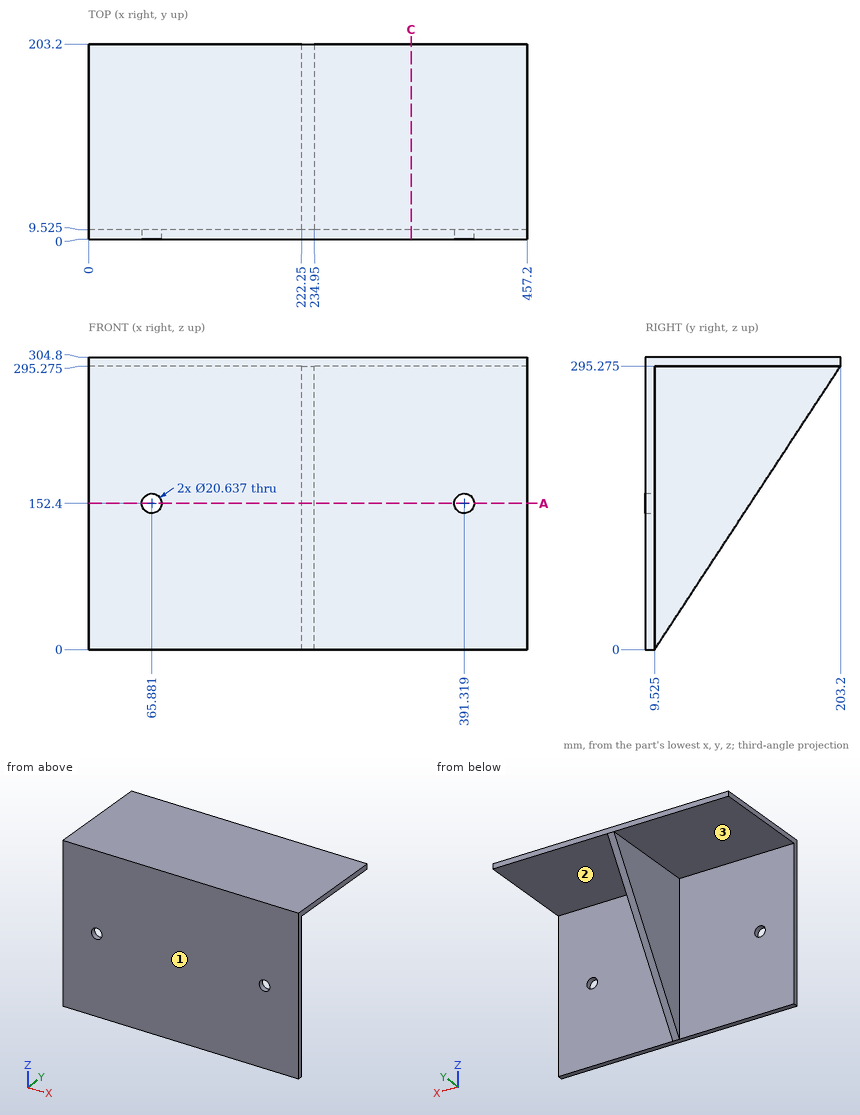
Verification items for this drawing (mm, ordinates from the low corner). A direction names the side the tool comes from. Give positions to 0.01 mm unless a question says otherwise; leave off trailing zeros. Order: outer loops, then holes, each group sorted by start corner. A loop starts at its lowest first (then second) coordinate and runs counter-clockwise, first axis right, second up.
1) Cross-section at A-A (z = 152.4). Give the number of separate pieces and of enclosed holes in the cut face, then the cut area to 3 significant figures.
Results are:
separate pieces: 3
enclosed holes: 0
area: 5,230 mm2
2) Material ranges on probe 1 along Y at (x, z) = (197, 51.5) (1 decimal); probe 2 along Z at (x, y) = (241, 108) (1 decimal); probe 3 along X at (y, z) = (100, 208.5), recorded low to high.
Results are:
probe 1: y = 0 to 9.5
probe 2: z = 295.3 to 304.8
probe 3: x = 222.25 to 234.95
3) Cross-section at C-C (x = 336). Record the boundary of the cut face in (y, z) (1 decimal).
Results are:
outline: (0, 0) - (9.5, 0) - (9.5, 295.3) - (203.2, 295.3) - (203.2, 304.8) - (0, 304.8) - close
4) Tool access check on the marked faces 1, 2 and 3. Record the directions out of +Z, -Z, +X, -X, +Y, -Y that give a thin tool (end or side, any length) a straight path to the whole face; none if there is none.
Results are:
face 1: +Z, -Z, +X, -X, -Y
face 2: -Z, +X, +Y
face 3: -Z, -X, +Y
5) Gauge pin test, flat ends, axial feed: pin 1 (1 mm diameter, centred on y = 95.5, z = 207, fed in from -X); pin 2 (23.5 mm diameter, centred on x = 65.88, z = 152.4, fed in from +Y) (1 decimal); pin 3 (8 mm diameter, centred on y = 37.5, z = 61, fed in from +X). Record the tip position at first contact, or that the pin passes through.
Results are:
pin 1: stops at x = 222.25
pin 2: stops at y = 9.5
pin 3: stops at x = 234.95
